```python
from build123d import *

# Parameters (mm, degrees)
ESQUISSE1_W        = 100
ESQUISSE1_H        = 100
ESQUISSE1_R        = 23.5
BOSS_EXTRU_1_DEPTH = 4.6


with BuildPart() as part:
    # Esquisse1 → Boss.-Extru.1 (new body)
    with BuildSketch(Plane.XY):
        with Locations((5.828319543, -13.849884125)):
            Rectangle(ESQUISSE1_W, ESQUISSE1_H)
        with Locations((5.828319543, -13.849884125)):
            Circle(ESQUISSE1_R, mode=Mode.SUBTRACT)
    extrude(amount=BOSS_EXTRU_1_DEPTH)


solid = part.part
```
Geometry check sheet. Reference: the model listing, model coordinates, mm. Coordinates: 2 decimals unless noted, no trailing zeros. Order: outer loops, then holes, each group sorted by start corner. A loop starts at its lowest first (then second) coordinate and runs counter-clockwise, first axis right, second up. Notation, with made-up numbers: (15.25, -33) - (70.25, -33) arc R17 ccw to (70.25, -12) - close; hole circle Ø10 at (-10.5, 52). An arc over 180 degrees is marked (long way). Answer in a Markdown table with one row per item. Add a question column.
1. Section check A-A (y = -28.5). Enter the section's corners in (x, z).
2. Section check C-C (z = 2.1). Enter the section's corners in (x, y).
3. Material ranges on L1, parallel to Y at x = 22.5, z = 1.85; L2, parallel to Y at x = 22, z = 1.6; L3, parallel to X at y = 7, z = 1.6, recorded low to high. Write a range as [from, to].
4. Draft check along Y on faces 1 (the face through (5, 36.15, 2)), 2 (the face through (-44.172, -15, 2)), 3 (the face through (0.73, -36.79, 2.27)). Enter one of: +Y half, -Y half, draft (parallel to the pull), parting line (faces both ways), or undercut.
5. Section check B-B (x = -7). Enter the section's corners in (y, z).
Data:
| question | item | result |
|---|---|---|
| 1 | outline | (-44.17, 0) - (-12.55, 0) - (-12.55, 4.6) - (-44.17, 4.6) - close; (24.2, 0) - (55.83, 0) - (55.83, 4.6) - (24.2, 4.6) - close |
| 2 | outline | (-44.17, -63.85) - (55.83, -63.85) - (55.83, 36.15) - (-44.17, 36.15) - close; hole circle Ø47 at (5.83, -13.85) |
| 3 | L1 | y = [-63.85, -30.41], [2.71, 36.15] |
| 3 | L2 | y = [-63.85, -30.9], [3.2, 36.15] |
| 3 | L3 | x = [-44.17, -5.01], [16.67, 55.83] |
| 4 | face 1 | +Y half |
| 4 | face 2 | draft |
| 4 | face 3 | undercut |
| 5 | outline | (-63.85, 0) - (-33.54, 0) - (-33.54, 4.6) - (-63.85, 4.6) - close; (5.84, 0) - (36.15, 0) - (36.15, 4.6) - (5.84, 4.6) - close |
